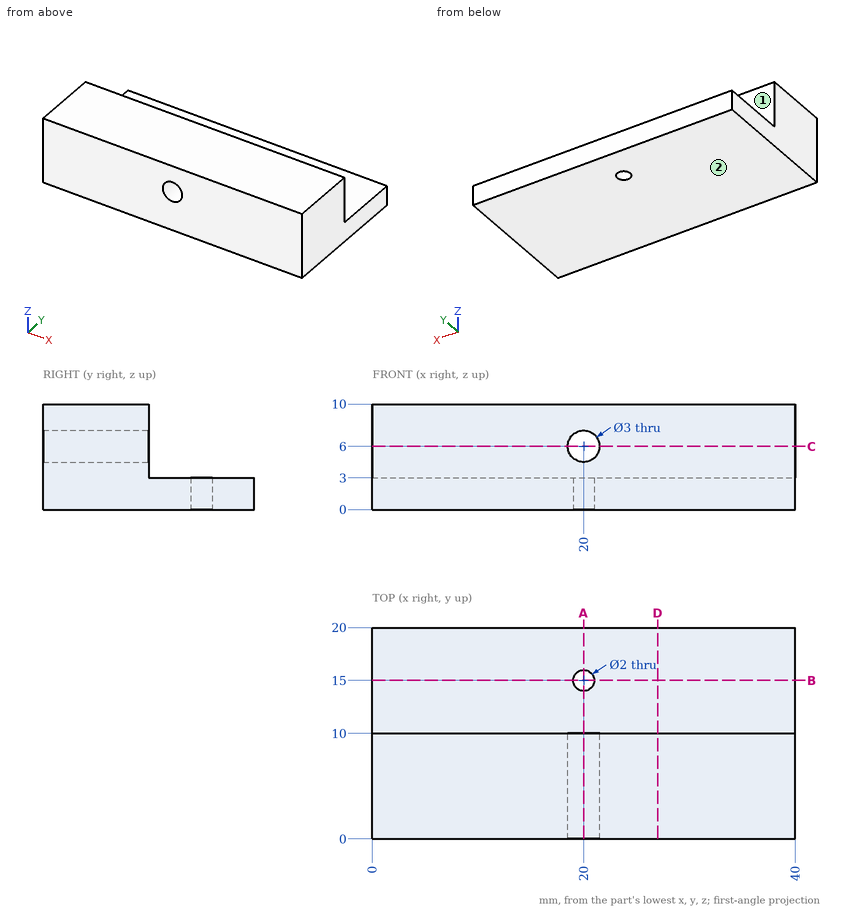
The figure shows three views and two pictorial views of one solid part (mm, origin at its lowest corner). Answer the questions. A direction names the side the tool comes from. Round coordinates to 2 decimals unless told otherwise and drop trailing zeros. Write each loop counter-clockwise with the first axis right and the second up, starting at its lowest first coordinate (ties: lowest second). Pieces come first, ordered by that corner, then holes. Notation, with made-up numbers: (49.5, 52.25) - (103.5, 52.25) arc R26 cw to (103.5, 73.25) - close; hole circle Ø11 at (13, -8.5). An arc over 180 degrees is marked (long way). Answer in a Markdown table with one row per item. Add a question column.
1. Given pin 1 (1.6 mm diameter, centred on x = 20, y = 15, fed in from -Z); pin 2 (3 mm diameter, centred on x = 25, z = 8, fed in from +Y); pin 3 (4 mm diameter, centred on x = 24.5, y = 13, fed in from +Z), each flat-ended and moving along its own axis, determine where each tip first touches the part or whether it passes through.
2. A cutting plane is placed at B-B, the plane y = 15. Determine the outline of the cut face in (x, z), and give its area (3 significant figures).
3. A cutting plane is placed at C-C, the plane z = 6. Determine the outline of the cut face in (x, y), and give its area (3 significant figures).
4. For the marked faces 1 and 2, determine the directions among +Z, -Z, +X, -X, +Y, -Y from which every point of the face is accessible in a straight line to the end or side of a thin tool.
5. A cutting plane is placed at D-D, the plane x = 27. Determine the outline of the cut face in (y, z).
6. Find the intervals of material crossed by line 1 along Y through (x, z) = (20, 1.15); line 2 along Z through (x, y) = (38, 18); line 3 along Y through (x, z) = (17, 6.5), in increasing order. Write a range as from..to.
7. A cutting plane is placed at A-A, the plane x = 20. Determine the outline of the cut face in (y, z), and give its area (3 significant figures).
Worked out:
| question | item | result |
|---|---|---|
| 1 | pin 1 | through |
| 1 | pin 2 | y = 10 |
| 1 | pin 3 | z = 3 |
| 2 | outline | (0, 0) - (19, 0) - (19, 3) - (0, 3) - close; (21, 0) - (40, 0) - (40, 3) - (21, 3) - close |
| 2 | area | 114 mm^2 |
| 3 | outline | (0, 0) - (18.5, 0) - (18.5, 10) - (0, 10) - close; (21.5, 0) - (40, 0) - (40, 10) - (21.5, 10) - close |
| 3 | area | 370 mm^2 |
| 4 | face 1 | +Z, +X, -X, +Y |
| 4 | face 2 | -Z, +X, -X, +Y, -Y |
| 5 | outline | (0, 0) - (20, 0) - (20, 3) - (10, 3) - (10, 10) - (0, 10) - close |
| 6 | line 1 | 0..14, 16..20 |
| 6 | line 2 | 0..3 |
| 6 | line 3 | 0..10 |
| 7 | outline | (0, 0) - (14, 0) - (14, 3) - (10, 3) - (10, 4.5) - (0, 4.5) - close; (0, 7.5) - (10, 7.5) - (10, 10) - (0, 10) - close; (16, 0) - (20, 0) - (20, 3) - (16, 3) - close |
| 7 | area | 94.0 mm^2 |
